Here's the drawing with two shaded views (mm, measured from the low corner). I have some questions. A direction names the side the tool comes from. Round coordinates to 2 decimals unless told otherwise and drop trailing zeros. Order: outer loops, then holes, each group sorted by start corner. A loop starts at its lowest first (then second) coordinate and runs counter-clockwise, first axis right, second up.
Q1. If we section it at C-C (y = 16): Please give me the cut outline in (x, z) (1 decimal).
Q2. Will these pins go through, and if not, where does the flat tip stop? P1, Ø4.5, axis at y = 43.66, z = 26.93, coming from the -X side; P2, Ø4, axis at x = 80, y = 21.5, coming from the +Z side.
Q3. For the marked faces 1 and 2, which set-ups out of +Z, -Z, +X, -X, +Y, -Y let a thin tool reach every point of the face, with its end or its side?
Q4. If I drill on line 1 (Y direction, x = 10, z = 46); line 2 (X direction, y = 73.5, z = 4.5) (1 decimal); line 3 (Z direction, x = 62, y = 23), over which ranges is the centre line in solid material (lowest first)?
Q5. If we section it at A-A (z = 40): Please give me the cut outline in (x, y) (1 decimal).
Q6. If we section it at B-B (x = 27.5): Please give me the cut outline in (y, z).
Q7. We'd pull the mould along X, two halves only. Please class the marked faces 3, 4 and 5: pulls with the +X half, pulls with the -X half, needs draft (parallel to the pull), parting line crosses it, or undercut.
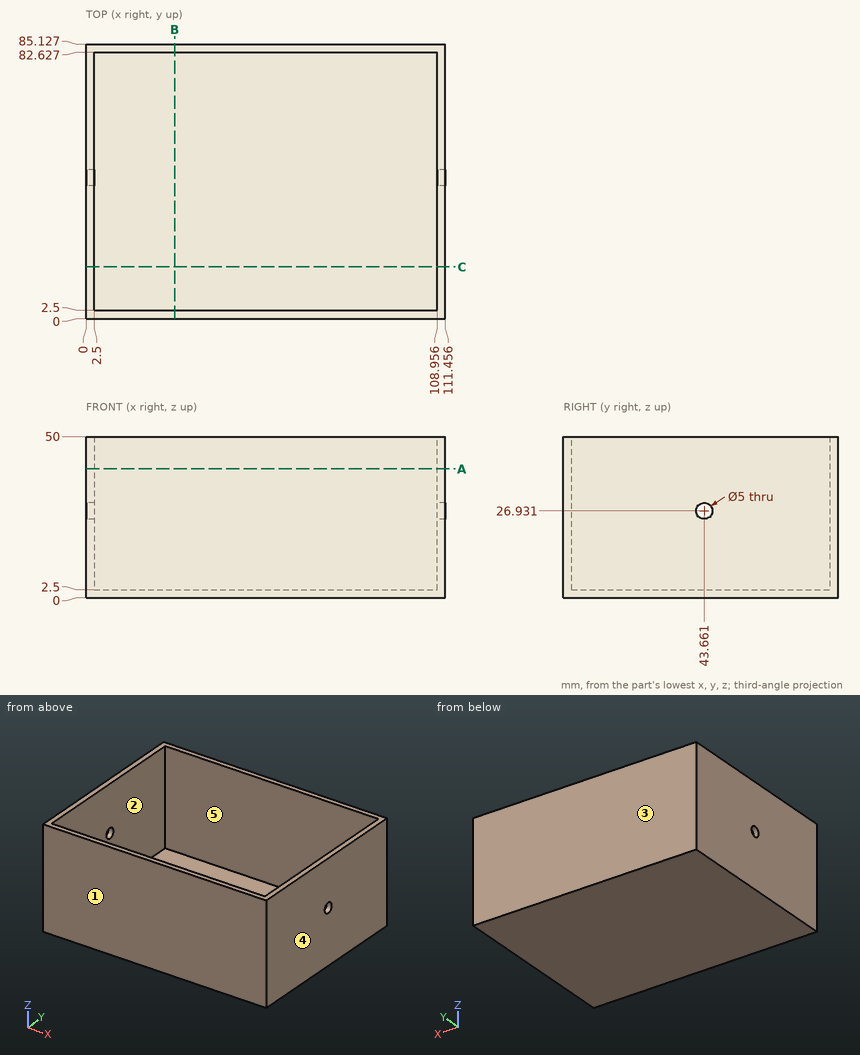
Solution:
1. outline: (0, 0) - (111.5, 0) - (111.5, 50) - (109, 50) - (109, 2.5) - (2.5, 2.5) - (2.5, 50) - (0, 50) - close
2. P1: passes through
2. P2: stops at z = 2.5
3. face 1: +Z, -Z, +X, -X, -Y
3. face 2: +Z
4. line 1: y = 0 to 2.5, 82.63 to 85.13
4. line 2: x = 0 to 2.5, 109 to 111.5
4. line 3: z = 0 to 2.5
5. outline: (0, 0) - (111.5, 0) - (111.5, 85.1) - (0, 85.1) - close; hole (2.5, 2.5) - (109, 2.5) - (109, 82.6) - (2.5, 82.6) - close
6. outline: (0, 0) - (85.13, 0) - (85.13, 50) - (82.63, 50) - (82.63, 2.5) - (2.5, 2.5) - (2.5, 50) - (0, 50) - close
7. face 3: needs draft
7. face 4: pulls with the +X half
7. face 5: undercut
